Read the model definition and answer for the solid it produces. Units are mm, in the model's axes. A direction names the side the tool comes from. Give positions to 0.01 mm unless a question says otherwise; leave off trailing zeros. Loops run counter-clockwise (first coordinate to the right, second up) from the corner with the lowest first, then second, coordinate; pieces in that order, holes last. Notation, with made-up numbers: (39.25, -15) - (59.25, -15) arc R24 ccw to (59.25, 0) - close; hole circle Ø1 at (55.5, 33). An arc over 180 degrees is marked (long way). Put each result on its own line as item: value. Start each with the question number.
1. For a pull along X with two mould halves and no side action, classify faces 3 (the flat face through (45, 4, 1)), 4 (the flat face through (-1, 0, -1)), 5 (the cylindrical face through (-29.045, 3.944, 10.443)) as released by +X, released by -X, zero draft, split by the parting line, or undercut.
2. A cutting plane is placed at C-C, the plane y = 6. Determine the outline of the cut face in (x, z), plus the area to 3 significant figures.
3. A cutting plane is placed at B-B, the plane z = 23.7. Determine the outline of the cut face in (x, y), plus the area to 3 significant figures.
4. For faces 1 (the cylindrical face through (35.27, 3.94, 24.92)), 2 (the flat face through (22, 2, 7)), determine the directions among +Z, -Z, +X, -X, +Y, -Y from which every point of the face is accessible in a straight line to the end or side of a thin tool.
5. A cutting plane is placed at A-A, the plane x = 18. Determine the outline of the cut face in (y, z).
6. Consider L1, parallel to Z at x = -20.5, y = 4.5; L2, parallel to X at y = 6, z = 23.7; L3, parallel to Z at x = 35, y = 5. Determine where each line is inside the solid, lowest interval first. Write a range as from..to.
7. A cutting plane is placed at D-D, the plane x = -35. Determine the outline of the cut face in (y, z).
```python
from build123d import *

# Parameters (mm, degrees)
SKETCH_1_W            = 90
SKETCH_1_H            = 100
EXTRUDE_1_DEPTH       = 8
M20X1_51_D            = 18.5
M25X1_51_D            = 23.5
SKETCH_6_W            = 8
SKETCH_6_H            = 8
CUT_EXTRUDE_1_DEPTH   = 4
FILLET_1_R            = 0.3
SKETCH_7_R            = 3.5
CUT_EXTRUDE_2_DEPTH   = 9
HOLE_WIZARD_M31_D     = 2.5
HOLE_WIZARD_M31_DEPTH = 8.5
HOLE_WIZARD_M31_TIP   = 0.751075774


with BuildPart() as part:
    # Эскиз1 → Бобышка-Вытянуть1 (new body)
    with BuildSketch(Plane(origin=(0, 0, 0), x_dir=(1, 0, 0), z_dir=(0, 1, 0))):
        Rectangle(SKETCH_1_W, SKETCH_1_H)
    extrude(amount=EXTRUDE_1_DEPTH)

    # Отверстие обработанное метчиком M20x1,51 (through all)
    with Locations(Plane(origin=(0, 8, 0), x_dir=(1, 0, 0), z_dir=(0, 1, 0))):
        with Locations((-20.5, 30.1), (18, 30.1), (-20.5, -6.9)):
            Hole(M20X1_51_D / 2)

    # Отверстие обработанное метчиком M25x1,51 (through all)
    with Locations(Plane(origin=(0, 8, 0), x_dir=(1, 0, 0), z_dir=(0, 1, 0))):
        with Locations((18, 30.1)):
            Hole(M25X1_51_D / 2)

    # Эскиз6 → Вырез-Вытянуть1 (cut)
    with BuildSketch(Plane.XZ):
        with Locations((18, 6.9)):
            Rectangle(SKETCH_6_W, SKETCH_6_H)
    extrude(amount=-CUT_EXTRUDE_1_DEPTH, mode=Mode.SUBTRACT)

    # Скругление1
    fillet_1_edges = [part.edges().sort_by_distance(p)[0] for p in [
        (14, 2, 2.9),
        (14, 2, 10.9),
        (22, 2, 10.9),
        (22, 2, 2.9),
    ]]
    fillet(fillet_1_edges, radius=FILLET_1_R)

    # Эскиз7 → Вырез-Вытянуть2 (cut)
    with BuildSketch(Plane.XZ.offset(-4)):
        with Locations(Location((18, 6.9, 0), (0, 0, 270))):
            Circle(SKETCH_7_R)
    extrude(amount=-CUT_EXTRUDE_2_DEPTH, mode=Mode.SUBTRACT)

    # Отверстие обработанное метчиком M31
    with Locations(Plane(origin=(0, 8, 0), x_dir=(1, 0, 0), z_dir=(0, 1, 0))):
        with Locations((35, -23.7), (-35, -23.7)):
            Hole(HOLE_WIZARD_M31_D / 2, depth=HOLE_WIZARD_M31_DEPTH)
            with Locations((0, 0, -(HOLE_WIZARD_M31_DEPTH + HOLE_WIZARD_M31_TIP / 2))):  # 118° drill point
                Cone(0, HOLE_WIZARD_M31_D / 2, HOLE_WIZARD_M31_TIP, mode=Mode.SUBTRACT)


solid = part.part
```
Return value:
1. face 3: released by +X
1. face 4: zero draft
1. face 5: undercut
2. outline: (-45, -50) - (45, -50) - (45, 50) - (-45, 50) - close; hole circle Ø2.5 at (-35, 23.7); hole circle Ø18.5 at (-20.5, -30.1); hole circle Ø18.5 at (-20.5, 6.9); hole circle Ø23.5 at (18, -30.1); hole circle Ø7 at (18, 6.9); hole circle Ø2.5 at (35, 23.7)
2. area: 7,980 mm2
3. outline: (-45, 0) - (-36.25, 0) - (-36.25, 8) - (-45, 8) - close; (-33.75, 0) - (33.75, 0) - (33.75, 8) - (-33.75, 8) - close; (36.25, 0) - (45, 0) - (45, 8) - (36.25, 8) - close
3. area: 680 mm2
4. face 1: +Y, -Y
4. face 2: -Y
5. outline: (0, -50) - (8, -50) - (8, -41.85) - (0, -41.85) - close; (0, -18.35) - (8, -18.35) - (8, 3.4) - (4, 3.4) - (4, 2.9) - (0, 2.9) - close; (0, 10.9) - (4, 10.9) - (4, 10.4) - (8, 10.4) - (8, 50) - (0, 50) - close
6. L1: z = -50..-39.35, -20.85..-2.35, 16.15..50
6. L2: x = -45..-36.25, -33.75..33.75, 36.25..45
6. L3: z = -50..22.45, 24.95..50
7. outline: (0, -50) - (8, -50) - (8, 22.45) - (0, 22.45) - close; (0, 24.95) - (8, 24.95) - (8, 50) - (0, 50) - close
